The listing builds one solid part. Answer for the finished solid, in the listing's coordinates (mm). Face numbers are marked on the shaded views. A direction names the side the tool comes from. Give positions to 0.01 mm unless a question says otherwise; leave off trailing zeros. Loops run counter-clockwise (first coordinate to the right, second up) from the corner with the lowest first, then second, coordinate; pieces in that order, holes last. Notation, with made-up numbers: (51.5, -34.5) -> (69.5, -34.5) arc R24 ccw to (69.5, -9.5) -> close; hole circle Ø4 at (-30, -12). An arc over 180 degrees is marked (long way). One line per question, with ' | ' between items. Start each with the question number.
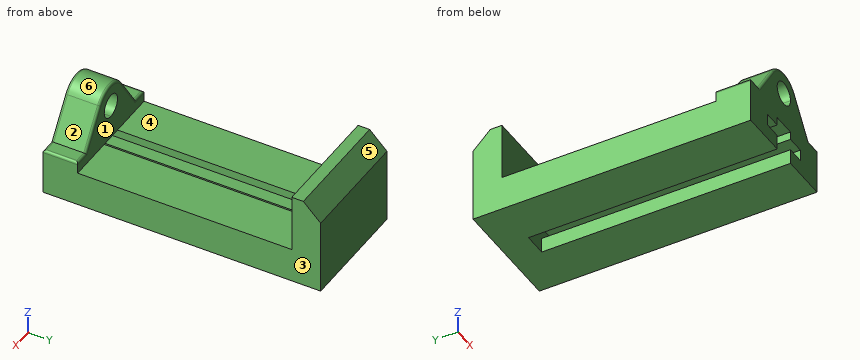
from build123d import *

# Parameters (mm, degrees)
F1_DEPTH  = 38.1
F3_DEPTH  = 273.05
F4_W      = 25.4
F4_H      = 38.1
F4_W_2    = 50.8
F5_DEPTH  = 12.7
F7_DEPTH  = 38.1
F8_R      = 2.54
F10_DEPTH = 63.5
F11_SIZE  = 19.05


with BuildPart() as f1:
    # F0 (on Top) → F1 (new body)
    with BuildSketch(Plane.XY):
        Polygon((-63.5, -152.4), (63.5, -152.4), (63.5, 152.4), (-63.5, 152.4), (-63.5, 114.3), (-63.5, 101.6), (-63.5, 88.9), align=None)
    extrude(amount=F1_DEPTH)

    # F2 (on face) → F3 (cut)
    with BuildSketch(Plane.XZ.offset(152.4)):
        Polygon((-12.7, 0), (0, 0), (12.7, 0), (12.7, 16.51), (31.75, 16.51), (31.75, 29.21), (12.7, 29.21), (12.7, 38.1), (-12.7, 38.1), (-12.7, 29.21), (-31.75, 29.21), (-31.75, 16.51), (-12.7, 16.51), align=None)
    extrude(amount=-F3_DEPTH, mode=Mode.SUBTRACT)

    # F4 (on face) → F5 (join)
    with BuildSketch(Plane.XY.offset(38.1)):
        with Locations((0, -133.35)):
            Rectangle(F4_W, F4_H)
        with Locations((-38.1, -133.35)):
            Rectangle(F4_W_2, F4_H)
        with Locations((38.1, -133.35)):
            Rectangle(F4_W_2, F4_H)
    extrude(amount=F5_DEPTH)

    # F6 (on face) → F7 (join)
    with BuildSketch(Plane.XZ.offset(152.4)):
        with BuildLine():
            Line((-47.625, 50.8), (0, 50.8))
            Line((0, 50.8), (47.625, 50.8))
            Line((47.625, 50.8), (21.0934256055, 90.3501730104))
            ThreePointArc((21.0934256055, 90.3501730104), (0, 101.6), (-21.0934256055, 90.3501730104))
            Line((-21.0934256055, 90.3501730104), (-47.625, 50.8))
        make_face()
        with BuildLine():
            ThreePointArc((12.7, 76.2), (8.9802561211, 67.2197438789), (0, 63.5))
            ThreePointArc((0, 63.5), (-8.9802561211, 85.1802561211), (12.7, 76.2))
        make_face(mode=Mode.SUBTRACT)
    extrude(amount=-F7_DEPTH)

    # F8
    f8_edges = [f1.edges().sort_by_distance(p)[0] for p in [
        (-55.5625, -152.4, 50.8),
        (55.5625, -152.4, 50.8),
        (34.359213, -152.4, 70.575087),
        (63.5, -133.35, 50.8),
        (-55.5625, -114.3, 50.8),
        (55.5625, -114.3, 50.8),
        (34.359213, -114.3, 70.575087),
        (0, -152.4, 101.6),
        (0, -114.3, 101.6),
        (-34.359213, -152.4, 70.575087),
        (-34.359213, -114.3, 70.575087),
        (-63.5, -133.35, 50.8),
    ]]
    fillet(f8_edges, radius=F8_R)

    # F9 (on face) → F10 (join)
    with BuildSketch(Plane.XY.offset(38.1)):
        Polygon((63.5, 152.4), (-63.5, 152.4), (-63.5, 120.65), (-12.7, 120.65), (12.7, 120.65), (63.5, 120.65), align=None)
    extrude(amount=F10_DEPTH)

    # F11
    f11_edges = [f1.edges().sort_by_distance(p)[0] for p in [
        (0, 152.4, 101.6),
    ]]
    chamfer(f11_edges, length=F11_SIZE)


solid = f1.part
1. Determine the mould class of the marked faces 4, 5 and 6 for opening direction Y: released by +Y, released by -Y, zero draft, split by the parting line, or undercut.
2. Straight lines are drawn through the part: L1, parallel to Y at x = 45.5, z = 43; L2, parallel to X at y = -93, z = 29; L3, parallel to Z at x = 30, y = -60. For each, find the intervals that lie inside material, in ascending order.
3. The part is cut by section B-B (x = -5). Count the separate pieces of the cut face and the enclosed holes in it, plus the area to 3 significant figures.
4. For the marked faces 1, 2 and 3, determine the directions among +Z, -Z, +X, -X, +Y, -Y from which every point of the face is accessible in a straight line to the end or side of a thin tool.
5. The part is cut by section A-A (y = -33.5). Write down the section's boundary in (x, z).
6. Each of these flat-tipped pins is pushed along its axis until it touches: pin 1 Ø10.5 at (x, y) = (52.5, -132) entering from +Z; pin 2 Ø6.5 at (x, y) = (-57, -139.5) entering from +Z; pin 3 Ø4 at (x, y) = (48.5, 104) entering from +Z. Where does it stop, or does it pass through?
Check sheet entries:
1) face 4: undercut | face 5: released by +Y | face 6: zero draft
2) L1: y = -152.4 to -114.3, 120.65 to 152.4 | L2: x = -63.5 to -31.75, 31.75 to 63.5 | L3: z = 0 to 16.51, 29.21 to 38.1
3) separate pieces: 3 | enclosed holes: 0 | area: 4,550 mm^2
4) face 1: +Z, +X, -X | face 2: +Z, +X, -Y | face 3: +Z, -Z, +X, +Y, -Y
5) outline: (-63.5, 0) -> (-12.7, 0) -> (-12.7, 16.51) -> (-31.75, 16.51) -> (-31.75, 29.21) -> (-12.7, 29.21) -> (-12.7, 38.1) -> (-63.5, 38.1) -> close; (12.7, 0) -> (63.5, 0) -> (63.5, 38.1) -> (12.7, 38.1) -> (12.7, 29.21) -> (31.75, 29.21) -> (31.75, 16.51) -> (12.7, 16.51) -> close
6) pin 1: stops at z = 51.36 | pin 2: stops at z = 50.8 | pin 3: stops at z = 38.1
